Here's how the part is built. I have some questions about the finished solid (model axes, mm). A direction names the side the tool comes from. Coordinates: 2 decimals unless noted, no trailing zeros. Order: outer loops, then holes, each group sorted by start corner. A loop starts at its lowest first (then second) coordinate and runs counter-clockwise, first axis right, second up. Notation, with made-up numbers: (32, 82.25) - (68, 82.25) arc R24 ccw to (68, 121.25) - close; hole circle Ø7 at (-26, 43.25). An arc over 180 degrees is marked (long way). Use one line per item in the form item = value. Start each with the question number.
from build123d import *

# Parameters (mm, degrees)
F0_W     = 67.757116
F0_H     = 66.861842
F1_DEPTH = 6.35
F2_W     = 27.674626
F2_H     = 25.4
F3_DEPTH = 17.78
F4_R     = 5.08
F5_R     = 5.08


with BuildPart() as f1:
    # F0 (on Top) → F1 (new body)
    with BuildSketch(Plane.XY):
        with Locations((-1.752707, -10.752427)):
            Rectangle(F0_W, F0_H)
    extrude(amount=F1_DEPTH)

    # F2 (on face) → F3 (join)
    with BuildSketch(Plane.XY.offset(6.35)):
        with Locations((-1.518216, -12.386003)):
            Rectangle(F2_W, F2_H)
    extrude(amount=F3_DEPTH)

    # F4
    f4_edges = [f1.edges().sort_by_distance(p)[0] for p in [
        (12.319097, -25.086003, 15.24),
        (-15.355529, -25.086003, 15.24),
        (-15.355529, 0.313997, 15.24),
        (12.319097, 0.313997, 15.24),
    ]]
    fillet(f4_edges, radius=F4_R)

    # F5
    f5_edges = [f1.edges().sort_by_distance(p)[0] for p in [
        (-1.518216, -25.086003, 24.13),
    ]]
    fillet(f5_edges, radius=F5_R)


solid = f1.part
1) Which directions (+Z, -Z, +X, -X, +Y, -Y) give clear straight access to the entire face, cutting with the end or side of a thin tool? Please do faces 1 (the flat face through (-2, 0.314, 13)), 2 (the cylindrical face through (-13.828, -1.135, 12.789)), 3 (the cylindrical face through (-13.828, -23.637, 12.789)), 4 (the cylindrical face through (10.79, -23.64, 12.79)), 5 (the flat face through (-2, 5, 6.35)).
2) For pin 1 (5 mm diameter, centred on x = 10.5, z = 9.5, fed in from +Y); pin 2 (4 mm diameter, centred on y = -17, z = 14, fed in from +X); pin 3 (1.5 mm diameter, centred on x = -16.5, y = -3.5, fed in from +Z), each with a flat end and sliding along its axis, tell me the tip position at first contact or that it passes through.
3) Suppose I cut it at B-B, the plane y = -6. List the corners of the cut face in (x, z) for me.
4) Suppose I cut it at D-D, the plane z = 20.5. List the corners of the cut face in (x, y) for me.
5) Suppose I cut it at A-A, the plane z = 16.25. List the corners of the cut face in (x, y) for me.
6) I need wall thicknesses on probe 1 along Z at (x, y) = (-26.5, -8); probe 2 along X at (y, z) = (-14, 11.75); probe 3 along X at (y, z) = (-5.5, 23). Which ranges of each line are inside material? Lowest first, please. Write a range as [from, to].
7) Suppose I cut it at C-C, the plane x = -2. List the corners of the cut face in (y, z) for me, then the cut area to 3 significant figures.
From the geometry:
q1.face_1 = +Z, +X, -X, +Y
q1.face_2 = +Z, -X, +Y
q1.face_3 = +Z, -X, -Y
q1.face_4 = +Z, +X, -Y
q1.face_5 = +Z
q2.pin_1 = 0.26
q2.pin_2 = 12.32
q2.pin_3 = 6.35
q3.outline = (-35.63, 0) - (32.13, 0) - (32.13, 6.35) - (12.32, 6.35) - (12.32, 19.05) arc R5.08 ccw to (7.24, 24.13) - (-10.28, 24.13) arc R5.08 ccw to (-15.36, 19.05) - (-15.36, 6.35) - (-35.63, 6.35) - close
q4.outline = (-15.14, -20.01) arc R4.87 ccw to (-10.28, -24.87) - (7.24, -24.87) arc R4.87 ccw to (12.11, -20.01) - (12.11, -4.77) arc R4.87 ccw to (7.24, 0.1) - (-10.28, 0.1) arc R4.87 ccw to (-15.14, -4.77) - close
q5.outline = (-15.36, -20.01) arc R5.08 ccw to (-10.28, -25.09) - (7.24, -25.09) arc R5.08 ccw to (12.32, -20.01) - (12.32, -4.77) arc R5.08 ccw to (7.24, 0.31) - (-10.28, 0.31) arc R5.08 ccw to (-15.36, -4.77) - close
q6.probe_1 = [0, 6.35]
q6.probe_2 = [-15.36, 12.32]
q6.probe_3 = [-13.47, 10.43]
q7.outline = (-44.18, 0) - (22.68, 0) - (22.68, 6.35) - (0.31, 6.35) - (0.31, 19.05) arc R5.08 ccw to (-4.77, 24.13) - (-20.01, 24.13) arc R5.08 ccw to (-25.09, 19.05) - (-25.09, 6.35) - (-44.18, 6.35) - close
q7.area = 865 mm2
